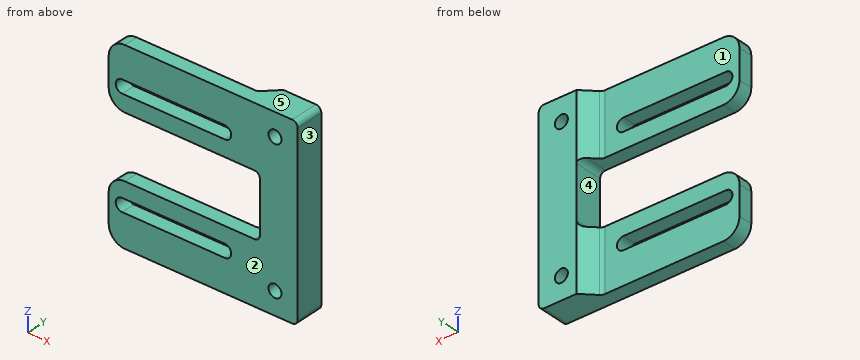
```python
from build123d import *

# Parameters (mm, degrees)
SKETCH1_W           = 7
SKETCH1_H           = 2.635
BOSS_EXTRUDE1_DEPTH = 17.2
CUT_EXTRUDE1_REACH  = 41.352
SKETCH2_R           = 1.2
CUT_EXTRUDE2_REACH  = 41.087
SKETCH3_W           = 28
SKETCH3_H           = 11.6
CHAMFER1_SIZE       = 2.635
FILLET2_R           = 1
FILLET3_R           = 3
FILLET4_R           = 1


with BuildPart() as part:
    # Sketch1 → Boss-Extrude1 (new, symmetric)
    with BuildSketch(Plane.XY):
        Polygon((0, -5.27), (0, -2.635), (-7, -2.635), (-35, -2.635), (-35, -5.27), align=None)
        with Locations((-3.5, -1.3175)):
            Rectangle(SKETCH1_W, SKETCH1_H)
    extrude(amount=BOSS_EXTRUDE1_DEPTH, both=True)

    # Sketch2 → Cut-Extrude1 (cut, up to next)
    with BuildSketch(Plane(origin=(0, 0, 0), x_dir=(1, 0, 0), z_dir=(0, 1, 0)), mode=Mode.PRIVATE) as cut_extrude1_sk1:
        with Locations(Location((-4.2, 13, 0), (0, 0, 270))):
            Circle(SKETCH2_R)
    cut_extrude1_tool1 = extrude(cut_extrude1_sk1.sketch, amount=-CUT_EXTRUDE1_REACH, mode=Mode.PRIVATE) & part.part
    # Sketch2 → Cut-Extrude1 (cut, up to next)
    with BuildSketch(Plane(origin=(0, 0, 0), x_dir=(1, 0, 0), z_dir=(0, 1, 0)), mode=Mode.PRIVATE) as cut_extrude1_sk2:
        with Locations(Location((-4.2, -13, 0), (0, 0, 270))):
            Circle(SKETCH2_R)
    cut_extrude1_tool2 = extrude(cut_extrude1_sk2.sketch, amount=-CUT_EXTRUDE1_REACH, mode=Mode.PRIVATE) & part.part
    add(cut_extrude1_tool1.solids().sort_by_distance((-4.2, 0, -13))[0], mode=Mode.SUBTRACT)
    add(cut_extrude1_tool2.solids().sort_by_distance((-4.2, 0, 13))[0], mode=Mode.SUBTRACT)

    # Sketch3 → Cut-Extrude2 (cut, up to next)
    with BuildSketch(Plane(origin=(0, -2.635, 0), x_dir=(1, 0, 0), z_dir=(0, 1, 0)), mode=Mode.PRIVATE) as cut_extrude2_sk1:
        with Locations((-21, 0)):
            Rectangle(SKETCH3_W, SKETCH3_H)
    cut_extrude2_tool1 = extrude(cut_extrude2_sk1.sketch, amount=-CUT_EXTRUDE2_REACH, mode=Mode.PRIVATE) & part.part
    # Sketch3 → Cut-Extrude2 (cut, up to next)
    with BuildSketch(Plane(origin=(0, -2.635, 0), x_dir=(1, 0, 0), z_dir=(0, 1, 0)), mode=Mode.PRIVATE) as cut_extrude2_sk2:
        with BuildLine():
            Line((-32.5, 11.2), (-13.5, 11.2))
            ThreePointArc((-13.5, 11.2), (-12.3, 10), (-13.5, 8.8))
            Line((-13.5, 8.8), (-32.5, 8.8))
            ThreePointArc((-32.5, 8.8), (-33.7, 10), (-32.5, 11.2))
        make_face()
    cut_extrude2_tool2 = extrude(cut_extrude2_sk2.sketch, amount=-CUT_EXTRUDE2_REACH, mode=Mode.PRIVATE) & part.part
    # Sketch3 → Cut-Extrude2 (cut, up to next)
    with BuildSketch(Plane(origin=(0, -2.635, 0), x_dir=(1, 0, 0), z_dir=(0, 1, 0)), mode=Mode.PRIVATE) as cut_extrude2_sk3:
        with BuildLine():
            Line((-32.5, -8.8), (-13.5, -8.8))
            ThreePointArc((-13.5, -8.8), (-12.3, -10), (-13.5, -11.2))
            Line((-13.5, -11.2), (-32.5, -11.2))
            ThreePointArc((-32.5, -11.2), (-33.7, -10), (-32.5, -8.8))
        make_face()
    cut_extrude2_tool3 = extrude(cut_extrude2_sk3.sketch, amount=-CUT_EXTRUDE2_REACH, mode=Mode.PRIVATE) & part.part
    add(cut_extrude2_tool1.solids().sort_by_distance((-21, -2.635, 0))[0], mode=Mode.SUBTRACT)
    add(cut_extrude2_tool2.solids().sort_by_distance((-23, -2.635, -10))[0], mode=Mode.SUBTRACT)
    add(cut_extrude2_tool3.solids().sort_by_distance((-23, -2.635, 10))[0], mode=Mode.SUBTRACT)

    # Chamfer1
    # the kernel refuses this chamfer: 2.635 mm, written as the material it adds along each edge
    with BuildSketch(Plane(origin=(-7, -2.635, 5.8), x_dir=(0.027495876610586358, 0.9996219169112968, 0), z_dir=(0, 0, 1))) as chamfer1_piece_1_section:
        Polygon((CHAMFER1_SIZE * 0.999621916911, CHAMFER1_SIZE * 0.0274958766106), (-CHAMFER1_SIZE * 0.0274958766106, CHAMFER1_SIZE * 0.999621916911), (0, 0), align=None)
    chamfer1_piece_1 = extrude(amount=11.4, mode=Mode.PRIVATE)
    chamfer1_piece_1 = split(chamfer1_piece_1, bisect_by=Plane(origin=(-7.870614947, 0, 11.5), z_dir=(0, -1, 0)), keep=Keep.TOP, mode=Mode.PRIVATE)
    add(chamfer1_piece_1)
    with BuildSketch(Plane(origin=(-7, -2.635, -17.2), x_dir=(0.027495876610586358, 0.9996219169112968, 0), z_dir=(0, 0, 1))) as chamfer1_piece_2_section:
        Polygon((CHAMFER1_SIZE * 0.999621916911, CHAMFER1_SIZE * 0.0274958766106), (-CHAMFER1_SIZE * 0.0274958766106, CHAMFER1_SIZE * 0.999621916911), (0, 0), align=None)
    chamfer1_piece_2 = extrude(amount=11.4, mode=Mode.PRIVATE)
    chamfer1_piece_2 = split(chamfer1_piece_2, bisect_by=Plane(origin=(-7.870614947, 0, -11.5), z_dir=(0, -1, 0)), keep=Keep.TOP, mode=Mode.PRIVATE)
    add(chamfer1_piece_2)

    # Fillet2
    fillet2_edges = [part.edges().sort_by_distance(p)[0] for p in [
        (-7, -2.635, -5.8),
        (-7, -2.635, 5.8),
        (-9.635, -2.635, 11.5),
        (-9.635, -2.635, -11.5),
    ]]
    fillet(fillet2_edges, radius=FILLET2_R)

    # Fillet3
    fillet3_edges = [part.edges().sort_by_distance(p)[0] for p in [
        (-35, -3.9525, -17.2),
        (-35, -3.9525, 17.2),
        (-35, -3.9525, 5.8),
        (-35, -3.9525, -5.8),
    ]]
    fillet(fillet3_edges, radius=FILLET3_R)

    # Fillet4
    fillet4_edges = [part.edges().sort_by_distance(p)[0] for p in [
        (0, -2.635, 17.2),
        (0, -2.635, -17.2),
    ]]
    fillet(fillet4_edges, radius=FILLET4_R)


solid = part.part
```
Verification items for the finished model (mm, model axes). Face numbers are marked on the shaded views. A direction names the side the tool comes from. Round coordinates to 2 decimals unless told otherwise and drop trailing zeros. Write each loop counter-clockwise with the first axis right and the second up, starting at its lowest first coordinate (ties: lowest second). Pieces come first, ordered by that corner, then holes.
1. Section check D-D on x = -14. Enter the section's corners in (y, z) (3 decimals), plus the area to 3 significant figures.
2. Section check B-B on y = -4.6. Enter the section's corners in (x, z), plus the area to 3 significant figures.
3. Gauge pin test, flat ends, axial feed: P1, Ø1.9, axis at x = -4.2, z = -13, coming from the +Y side; P2, Ø1.6, axis at y = -2.5, z = -0.5, coming from the -X side; P3, Ø9, axis at x = -19.5, z = 9, coming from the +Y side (3 decimals). Record the tip position at first contact, or that the pin passes through.
4. Draft check along Z on the marked faces 3, 4 and 5. Enter one of: +Z half, -Z half, draft (parallel to the pull), parting line (faces both ways), or undercut.
5. Scan lines: L1, parallel to Z at x = -25, y = -3.1; L2, parallel to Z at x = -3.5, y = -1.2; L3, parallel to Y at x = -32, z = -14.5 (3 decimals). Record each from-to range of solid material in increasing order.
6. Section check A-A on z = 10. Enter the section's corners in (x, y) (3 decimals), plus the area to 3 significant figures.
7. Access from +Z, -Z, +X, -X, +Y, -Y to the whole of each face (thin tool, end or side, straight path). Record for the marked faces 1 and 2.
8. Section check C-C on x = -4.2. Enter the section's corners in (y, z), plus the area to 3 significant figures.
Answer:
1. outline: (-5.27, -17.2) - (-2.635, -17.2) - (-2.635, -11.2) - (-5.27, -11.2) - close; (-5.27, -8.8) - (-2.635, -8.8) - (-2.635, -5.8) - (-5.27, -5.8) - close; (-5.27, 5.8) - (-2.635, 5.8) - (-2.635, 8.8) - (-5.27, 8.8) - close; (-5.27, 11.2) - (-2.635, 11.2) - (-2.635, 17.2) - (-5.27, 17.2) - close
1. area: 47.4 mm2
2. outline: (-35, -14.2) arc R3 ccw to (-32, -17.2) - (-1, -17.2) arc R1 ccw to (0, -16.2) - (0, 16.2) arc R1 ccw to (-1, 17.2) - (-32, 17.2) arc R3 ccw to (-35, 14.2) - (-35, 8.8) arc R3 ccw to (-32, 5.8) - (-8, 5.8) arc R1 cw to (-7, 4.8) - (-7, -4.8) arc R1 cw to (-8, -5.8) - (-32, -5.8) arc R3 ccw to (-35, -8.8) - close; hole (-32.5, -11.2) - (-13.5, -11.2) arc R1.2 ccw to (-13.5, -8.8) - (-32.5, -8.8) arc R1.2 ccw to start; hole (-32.5, 8.8) - (-13.5, 8.8) arc R1.2 ccw to (-13.5, 11.2) - (-32.5, 11.2) arc R1.2 ccw to start; hole circle Ø2.4 at (-4.2, -13); hole circle Ø2.4 at (-4.2, 13)
2. area: 762 mm2
3. P1: passes through
3. P2: stops at x = -7
3. P3: stops at y = -2.635
4. face 3: draft
4. face 4: undercut
4. face 5: +Z half
5. L1: z = -17.2 to -11.2, -8.8 to -5.8, 5.8 to 8.8, 11.2 to 17.2
5. L2: z = -17.2 to -13.97, -12.03 to 12.03, 13.97 to 17.2
5. L3: y = -5.27 to -2.635
6. outline: (-35, -5.27) - (-33.7, -5.27) - (-33.7, -2.635) - (-35, -2.635) - close; (-12.3, -5.27) - (0, -5.27) - (0, 0) - (-7, 0) - (-9.342, -2.342) arc R1 cw to (-10.049, -2.635) - (-12.3, -2.635) - close
6. area: 57.8 mm2
7. face 1: +Z, -Z, -X, +Y
7. face 2: +Z, -Z, +X, -X, -Y
8. outline: (-5.27, -17.2) - (0, -17.2) - (0, -14.2) - (-5.27, -14.2) - close; (-5.27, -11.8) - (0, -11.8) - (0, 11.8) - (-5.27, 11.8) - close; (-5.27, 14.2) - (0, 14.2) - (0, 17.2) - (-5.27, 17.2) - close
8. area: 156 mm2
